Source: CAD feature listing. Evaluate the final solid. Frame: model axes, mm. A direction names the side the tool comes from. Round coordinates to 2 decimals unless told otherwise and drop trailing zeros. Loops run counter-clockwise (first coordinate to the right, second up) from the corner with the lowest first, then second, coordinate; pieces in that order, holes last. Notation, with made-up numbers: M -19,73.5 L 36,73.5 A25 cw 36,90.5 Z; hole C -27.75,78.5 d8. An arc over 180 degrees is marked long. One line per item, written item: value.
from build123d import *

# Parameters (mm, degrees)
PAD_DEPTH       = 4
FILLET_R        = 1.5
FILLET001_R     = 1
SKETCH003_R     = 1.5
PAD003_DEPTH    = 2
FILLET002_R     = 2
SKETCH004_W     = 6
SKETCH004_H     = 15
PAD004_DEPTH    = 6
SKETCH005_R     = 2
POCKET_DEPTH    = 21.984954
FILLET003_R     = 2.9
SKETCH006_R     = 2
POCKET001_DEPTH = 4.001


with BuildPart() as part:
    # Sketch → Pad (new body)
    with BuildSketch(Plane.XY):
        Polygon((0, 6), (-45, 6), (-45, -6), (0, -6), (30, -15), (30, 15), align=None)
    extrude(amount=PAD_DEPTH)

    # Fillet
    fillet_edges = [part.edges().sort_by_distance(p)[0] for p in [
        (30, 15, 2),
        (30, -15, 2),
    ]]
    fillet(fillet_edges, radius=FILLET_R)

    # Fillet001
    fillet001_edges = [part.edges().sort_by_distance(p)[0] for p in [
        (14.034489, 10.210347, 4),
        (14.034489, 10.210347, 0),
        (29.395396, 14.187393, 0),
        (29.395396, 14.187393, 4),
        (30, 0, 4),
        (30, 0, 0),
        (14.034489, -10.210347, 4),
        (14.034489, -10.210347, 0),
        (29.395396, -14.187393, 0),
        (29.395396, -14.187393, 4),
    ]]
    fillet(fillet001_edges, radius=FILLET001_R)

    # Sketch003 → Pad003 (join)
    with BuildSketch(Plane.XY.offset(3.5)):
        with Locations((-21, 0)):
            Circle(SKETCH003_R)
    extrude(amount=PAD003_DEPTH)

    # Fillet002
    fillet002_edges = [part.edges().sort_by_distance(p)[0] for p in [
        (-45, 0, 0),
    ]]
    fillet(fillet002_edges, radius=FILLET002_R)

    # Sketch004 (on Face6 of Fillet002) → Pad004 (join)
    with BuildSketch(Plane.XY.offset(4)):
        with Locations((-42, 0)):
            Rectangle(SKETCH004_W, SKETCH004_H)
    extrude(amount=PAD004_DEPTH)

    # Sketch005 (on Face17 of Pad004) → Pocket (cut, through all)
    with BuildSketch(Plane.XZ.offset(7.5)):
        with Locations((-42, 7)):
            Circle(SKETCH005_R)
    extrude(amount=-POCKET_DEPTH, mode=Mode.SUBTRACT)

    # Fillet003
    fillet003_edges = [part.edges().sort_by_distance(p)[0] for p in [
        (-45, 0, 10),
        (-39, 0, 10),
        (-45, -6.75, 4),
        (-39, -6.75, 4),
        (-45, 6.75, 4),
        (-39, 6.75, 4),
    ]]
    fillet(fillet003_edges, radius=FILLET003_R)

    # Sketch006 (on Face8 of Fillet003) → Pocket001 (cut, through all)
    with BuildSketch(Plane.XY.offset(4)):
        with Locations((-14, 0)):
            Circle(SKETCH006_R)
    extrude(amount=-POCKET001_DEPTH, mode=Mode.SUBTRACT)


solid = part.part
1. Section query A-A (y = 0). Return the cut outline in (x, z).
Report:
outline: M -45,2 A2 ccw -43,0 L -16,0 L -16,4 L -19.5,4 L -19.5,5.5 L -22.5,5.5 L -22.5,4 L -39,4 L -39,7.1 A2.9 ccw -41.9,10 L -42.1,10 A2.9 ccw -45,7.1 Z; M -12,0 L 29,0 A1 ccw 30,1 L 30,3 A1 ccw 29,4 L -12,4 Z; hole C -42,7 d4
2. Ray query, line 1 (Y direction, x = -14, z = 1.5); line 2 (Z direction, x = -30, y = 0.25); line 3 (Y direction, x = -7.5, z = 2). Return the intervals inside material, ascending. Write a range as [from, to].
Report:
line 1: y = [-6, -2], [2, 6]
line 2: z = [0, 4]
line 3: y = [-6, 6]
3. Section query C-C (y = -4.25). Return the cut outline in (x, z), and give its area (3 significant figures).
Report:
outline: M -45,2 A2 ccw -43,0 L 29,0 A1 ccw 30,1 L 30,3 A1 ccw 29,4 L -39,4 L -39,7.1 A2.9 ccw -41.9,10 L -42.1,10 A2.9 ccw -45,7.1 Z; hole C -42,7 d4
area: 319 mm2
4. Pin query (flat end, axial travel): pin 1 (6 mm diameter, centred on x = -7, z = 4.5, fed in from -Y); pin 2 (4.5 mm diameter, centred on x = -14, y = 0, fed in from +Z); pin 3 (6 mm diameter, centred on x = 1, z = 6.5, fed in from -Y); pin 4 (3 mm diameter, centred on x = -42, z = 7, fed in from +Y). Return the tip coordinate at first contact, or that it passes through.
Report:
pin 1: stops at y = -6
pin 2: stops at z = 4
pin 3: stops at y = -6.33
pin 4: passes through
5. Pull-direction query (Y, two-part tool) for faces 1 (the face through (14.317, -9.981, 0.285)), 2 (the face through (-15.6, -1.2, 2)), 3 (the face through (-39, 0, 6)), 4 (the face through (13.924, 9.863, 0.285)); classes: released by +Y, released by -Y, zero draft, split by the parting line, or undercut.
Report:
face 1: released by -Y
face 2: undercut
face 3: zero draft
face 4: released by +Y
6. Section query B-B (x = -14). Return the cut outline in (y, z), and give its area (3 significant figures).
Report:
outline: M -6,0 L -2,0 L -2,4 L -6,4 Z; M 2,0 L 6,0 L 6,4 L 2,4 Z
area: 32.0 mm2
7. Reachability of faces 5 (the face through (-44.2, -6.7, 4.9)), 6 (the face through (-21, 0, 5.5)), 7 (the face through (-22.5, 0.07, 4.74)) from +Z, -Z, +X, -X, +Y, -Y: full face, straight path, thin tool, end or side. Return the list, or none.
Report:
face 5: -Z, -X, -Y
face 6: +Z, +X, +Y, -Y
face 7: +Z
8. Section query D-D (z = 6.25). Return the cut outline in (x, y), and give its area (3 significant figures).
Report:
outline: M -45,-6 L -44.93,-6 L -44.93,-7.5 L -43.85,-7.5 L -43.85,7.5 L -44.93,7.5 L -44.93,6 L -45,6 Z; M -40.15,-7.5 L -39.07,-7.5 L -39.07,-6 L -39,-6 L -39,6 L -39.07,6 L -39.07,7.5 L -40.15,7.5 Z
area: 33.9 mm2
